from build123d import *

# Parameters (mm, degrees)
F0_W      = 60
F0_H      = 60
F1_DEPTH  = 6
F2_W      = 5
F2_H      = 5
F4_W      = 5
F4_H      = 5
F7_W      = 5
F7_H      = 5
F6_W      = 5
F6_H      = 5
F9_W      = 5
F9_H      = 5
F10_W     = 5
F10_H     = 5
F12_W     = 5
F12_H     = 5
F13_W     = 5
F13_H     = 5
F15_W     = 2.5
F15_H     = 5
F16_DEPTH = 55


with BuildPart() as f1:
    # F0 (on Top) → F1 (new body)
    with BuildSketch(Plane.XY):
        Rectangle(F0_W, F0_H)
    extrude(amount=F1_DEPTH)

    # F2 (on face) → F5 section 0
    with BuildSketch(Plane(origin=(0, 0, 0), x_dir=(1, 0, 0), z_dir=(0, 0, -1))):
        with Locations((-22.5, -22.5)):
            Rectangle(F2_W, F2_H)
    # F4 (on offset) → F5 section 1
    with BuildSketch(Plane.XY.offset(-80)):
        with Locations((-30, 30)):
            Rectangle(F4_W, F4_H)
    loft()

    # F7 (on offset) → F8 section 0
    with BuildSketch(Plane.XY.offset(-80)):
        with Locations((-30, -30)):
            Rectangle(F7_W, F7_H)
    # F6 (on face) → F8 section 1
    with BuildSketch(Plane(origin=(0, 0, 0), x_dir=(1, 0, 0), z_dir=(0, 0, -1))):
        with Locations((-22.5, 22.5)):
            Rectangle(F6_W, F6_H)
    loft()

    # F9 (on offset) → F11 section 0
    with BuildSketch(Plane.XY.offset(-80)):
        with Locations((30, -30)):
            Rectangle(F9_W, F9_H)
    # F10 (on face) → F11 section 1
    with BuildSketch(Plane(origin=(0, 0, 0), x_dir=(1, 0, 0), z_dir=(0, 0, -1))):
        with Locations((22.5, 22.5)):
            Rectangle(F10_W, F10_H)
    loft()

    # F12 (on offset) → F14 section 0
    with BuildSketch(Plane.XY.offset(-80)):
        with Locations((30, 30)):
            Rectangle(F12_W, F12_H)
    # F13 (on face) → F14 section 1
    with BuildSketch(Plane(origin=(0, 0, 0), x_dir=(1, 0, 0), z_dir=(0, 0, -1))):
        with Locations((22.5, -22.5)):
            Rectangle(F13_W, F13_H)
    loft()

    # F15 (on face) → F16 (join)
    with BuildSketch(Plane(origin=(0, 19.82575, 1.858664), x_dir=(1, 0, 0), z_dir=(0, -0.995634, -0.093341))):
        with Locations((-28.75, -69.717608)):
            Rectangle(F15_W, F15_H)
    extrude(amount=F16_DEPTH)


solid = f1.part
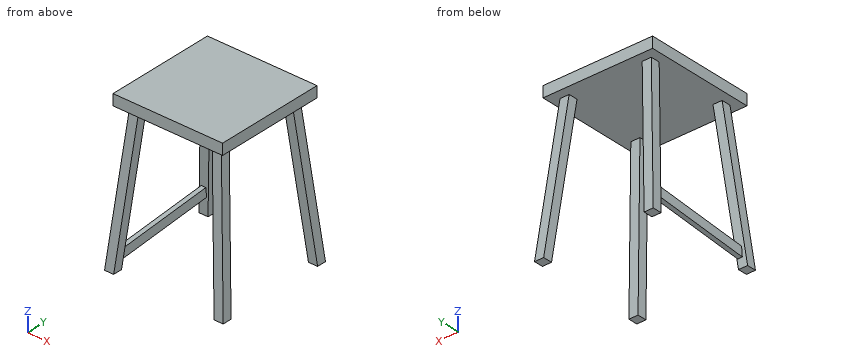
Can you work these out from the model? Positions are in its coordinate system, mm. Give positions to 0.01 mm unless a question says otherwise; leave off trailing zeros. Order: outer loops, then holes, each group sorted by start corner. A loop starts at its lowest first (then second) coordinate and runs counter-clockwise, first axis right, second up. Notation, with made-up numbers: M 86.5,-16.75 L 144.5,-16.75 A35 cw 144.5,15.25 Z; hole C 63.25,19 d6. An arc over 180 degrees is marked long. Use one line per item in the form item = value.
Item 1: Will these pins go through, and if not, where does the flat tip stop? pin 1 Ø3 at (y, z) = (13, -71) entering from +X; pin 2 Ø1.8 at (y, z) = (-5, 3) entering from +X; pin 3 Ø5 at (x, y) = (-6.5, 12) entering from -Z.
Values follow:
pin_1 = -27.5
pin_2 = 30
pin_3 = 0
Item 2: If we section it at A-A, the plane y = 1.5: Write out the boundary of the cut face in (x, z), and give its area (3 significant figures).
Values follow:
outline = M -30,-72.39 L -27.5,-72.39 L -27.5,-67.37 L -30,-67.37 Z; M -30,0 L 30,0 L 30,6 L -30,6 Z
area = 373 mm^2
Item 3: If we section it at C-C, the plane z = -15: Count the separate pieces of the cut face and the enclosed holes in it, and give its area (3 significant figures).
Values follow:
separate_pieces = 4
enclosed_holes = 0
area = 100 mm^2
Item 4: If I drill on line 1 along Z through (x, y) = (-1, -28); line 2 along X through (y, z) = (-23, -70.5); line 3 along Y through (x, z) = (28, -71), over which ranges is the centre line in solid material (lowest first)? Write a range as [from, to].
Values follow:
line_1 = [0, 6]
line_2 = [-30, -27.5]
line_3 = [-31.66, -26.66], [26.66, 31.66]
Item 5: If we section it at B-B, the plane x = 8: Write out the boundary of the cut face in (y, z), and give its area (3 significant figures).
Values follow:
outline = M -30,0 L 30,0 L 30,6 L -30,6 Z
area = 360 mm^2
